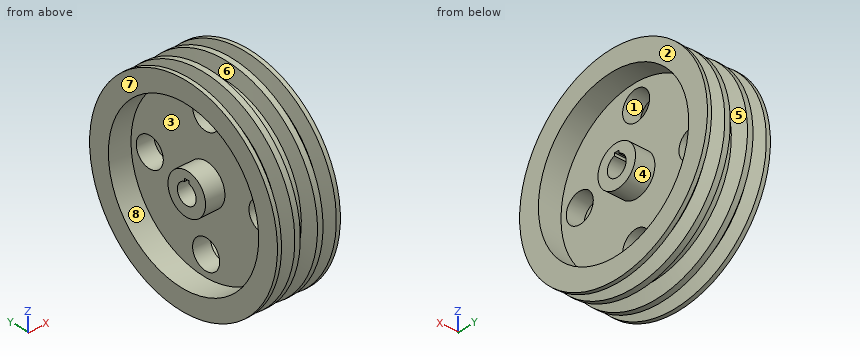
from build123d import *

# Parameters (mm, degrees)
CUT_EXTRUDE1_DEPTH      = 184.711730709
CUT_EXTRUDE1_DEPTH_BACK = 184.711730709
SKETCH2_R               = 18


with BuildPart() as part:
    # Sketch1 → Revolve2 (revolve)
    with BuildSketch(Plane.XY, mode=Mode.PRIVATE) as revolve2_sk:
        Polygon((17.448535783, 125), (20.724267892, 107), (30.724267892, 107), (34, 125), (39, 125), (39, 100), (11, 100), (11, 25), (35, 25), (35, 12.5), (0, 12.5), (-35, 12.5), (-35, 25), (-11, 25), (-11, 100), (-39, 100), (-39, 125), (-34, 125), (-30.724267892, 107), (-20.724267892, 107), (-17.448535783, 125), (-10.611364858, 125), (-7.33563275, 107), (7.33563275, 107), (10.611364858, 125), align=None)
    revolve(revolve2_sk.sketch.rotate(Axis((-121.58529461, 0, 0), (1, 0, 0)), 90), axis=Axis((-121.58529461, 0, 0), (1, 0, 0)))

    # Sketch2 → Cut-Extrude1 (cut, two sides: drawn at the far end of the back side and taken through both)
    with BuildSketch(Plane.ZY.offset(11).offset(-CUT_EXTRUDE1_DEPTH_BACK)):
        with Locations(Location((0, 75, 0), (0, 0, 180))):
            Circle(SKETCH2_R)
        with Locations(Location((75, 0, 0), (0, 0, 180))):
            Circle(SKETCH2_R)
        with Locations(Location((0, -75, 0), (0, 0, 180))):
            Circle(SKETCH2_R)
        with Locations(Location((-75, 0, 0), (0, 0, 180))):
            Circle(SKETCH2_R)
        with BuildLine():
            Line((15.5, -3), (15.5, 3))
            Line((15.5, 3), (12.1346611, 3))
            ThreePointArc((12.1346611, 3), (-12.5, 0), (12.1346611, -3))
            Line((12.1346611, -3), (15.5, -3))
        make_face()
    extrude(amount=CUT_EXTRUDE1_DEPTH + CUT_EXTRUDE1_DEPTH_BACK, mode=Mode.SUBTRACT)


solid = part.part
Could you check a few things on this model? Use its own coordinates, in mm. Face numbers are marked on the shaded views. A direction names the side the tool comes from. Round coordinates to 2 decimals unless told otherwise and drop trailing zeros.
(1) Imagine slicing it at A-A (y = 0). Count the separate pieces of the cut face and the enclosed holes in it, plus the area to 3 significant figures.
Response values:
separate pieces: 4
enclosed holes: 0
area: 5,550 mm2
(2) Which directions (+Z, -Z, +X, -X, +Y, -Y) give clear straight access to the entire face, cutting with the end or side of a thin tool? Please do the marked faces 1, 2, 3, 4 and 5.
Response values:
face 1: +X, -X
face 2: +Z, -Z, +X, +Y, -Y
face 3: -X
face 4: +X
face 5: none
(3) Please list where these lines run through material, in increasing order: line 1 along Y through (x, z) = (-3, 0); line 2 along Z through (x, y) = (27, 7.5); line 3 along Y through (x, z) = (28, 0).
Response values:
line 1: y = -107 to -93, -57 to -12.5, 12.5 to 57, 93 to 107
line 2: z = -106.74 to -99.72, -23.85 to -10, 10 to 23.85, 99.72 to 106.74
line 3: y = -107 to -100, -25 to -12.5, 12.5 to 25, 100 to 107
(4) If we mould it in two halves opening along X, with no side actions, what happens to the marked faces 6, 7 and 8? For each: released by +X, released by -X, zero draft, split by the parting line, or undercut.
Response values:
face 6: undercut
face 7: released by -X
face 8: zero draft
(5) I'm going to push flat-ended pins straight in: pin 1 (25 mm diameter, centred on y = 4.5, z = 0, fed in from -X); pin 2 (1 mm diameter, centred on x = -23, y = -51.5, fed in from +Z); pin 3 (1.8 mm diameter, centred on x = -2, y = -1, fed in from -Z). Where does each tip first touch, or does it pass through?
Response values:
pin 1: stops at x = -35
pin 2: stops at z = 94.06
pin 3: stops at z = -107
